Check sheet for the drawn part. Datum: minimum x, y, z corner. Units: mm. Round coordinates to 2 decimals unless told otherwise and drop trailing zeros. Order: outer loops, then holes, each group sorted by start corner. A loop starts at its lowest first (then second) coordinate and runs counter-clockwise, first axis right, second up. Notation, with made-up numbers: (-27, 49) -> (11, 49) arc R20 cw to (11, 66) -> close; hole circle Ø5 at (-29.5, 48). An arc over 180 degrees is marked (long way). Answer as a JSON object with one key per item and string values. Group by question number.
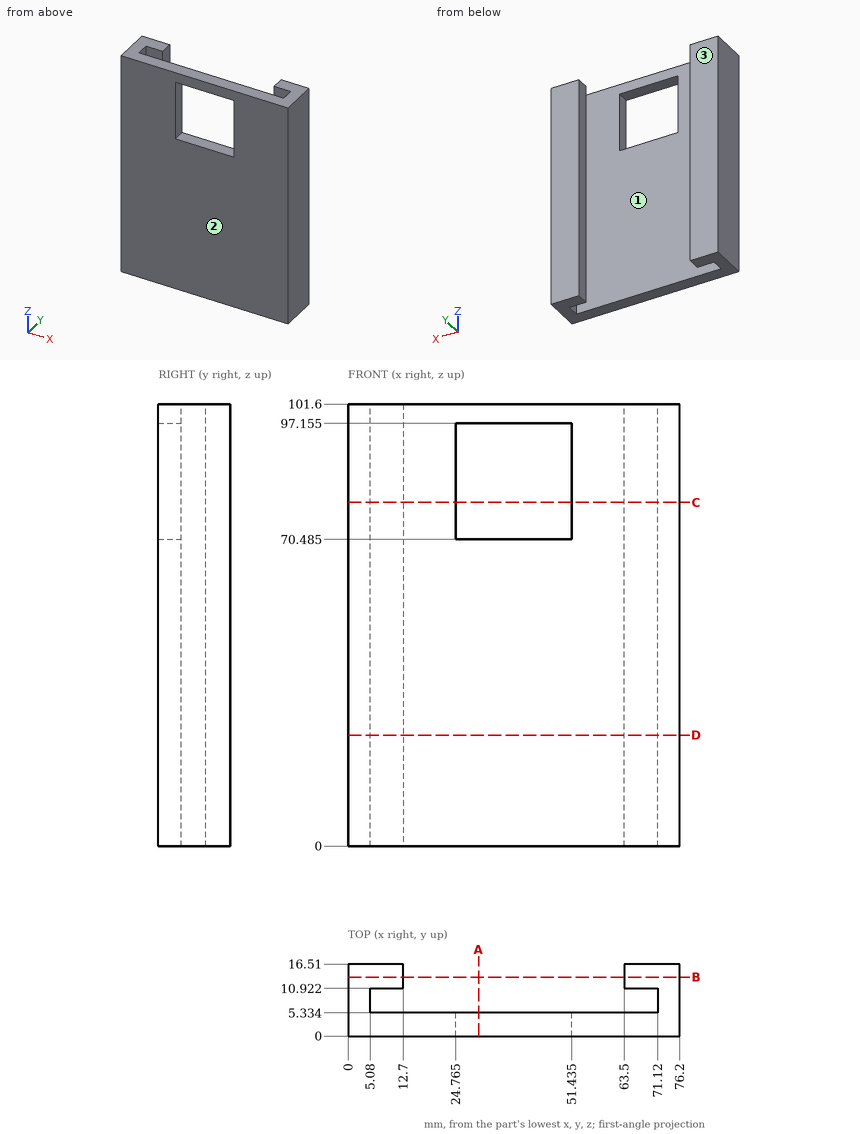
Item 1: Sectioned sample at D-D, the plane z = 25.5. Enter the section's corners in (x, y).
Item 2: Sectioned sample at A-A, the plane x = 30. Enter the section's corners in (y, z) (3 decimals).
Item 3: Depth check by flat-ended pin: pin 1 Ø1.5 at (x, y) = (14.5, 6.5) entering from +Z. Enter the tip coordinate at first touch or a pass-through.
Item 4: Mould release check, pull along Y, two halves, no side actions. Record for the marked faces 1, 2 and 3: pulls with the +Y half, pulls with the -Y half, needs draft (parallel to the pull), parting line crosses it, or undercut.
Item 5: Thickness scan on L1, parallel to X at y = 10.75, z = 73; L2, parallel to X at y = 15.5, z = 91; L3, parallel to Z at x = 27, y = 0.75 (3 decimals). Record the ranges inside material, lowest first.
Item 6: Sectioned sample at C-C, the plane z = 79. Enter the section's corners in (x, y) (3 decimals), then the cut area to 3 significant figures.
Item 7: Sectioned sample at B-B, the plane y = 13.5. Enter the section's corners in (x, z).
Result:
{
 "1": {"outline": "(0, 0) -> (76.2, 0) -> (76.2, 16.51) -> (63.5, 16.51) -> (63.5, 10.92) -> (71.12, 10.92) -> (71.12, 5.33) -> (5.08, 5.33) -> (5.08, 10.92) -> (12.7, 10.92) -> (12.7, 16.51) -> (0, 16.51) -> close"},
 "2": {"outline": "(0, 0) -> (5.334, 0) -> (5.334, 70.485) -> (0, 70.485) -> close; (0, 97.155) -> (5.334, 97.155) -> (5.334, 101.6) -> (0, 101.6) -> close"},
 "3": {"pin 1": "passes through"},
 "4": {"face 1": "undercut", "face 2": "pulls with the -Y half", "face 3": "pulls with the +Y half"},
 "5": {"L1": "x = 0 to 5.08, 71.12 to 76.2", "L2": "x = 0 to 12.7, 63.5 to 76.2", "L3": "z = 0 to 70.485, 97.155 to 101.6"},
 "6": {"outline": "(0, 0) -> (24.765, 0) -> (24.765, 5.334) -> (5.08, 5.334) -> (5.08, 10.922) -> (12.7, 10.922) -> (12.7, 16.51) -> (0, 16.51) -> close; (51.435, 0) -> (76.2, 0) -> (76.2, 16.51) -> (63.5, 16.51) -> (63.5, 10.922) -> (71.12, 10.922) -> (71.12, 5.334) -> (51.435, 5.334) -> close", "area": "463 mm2"},
 "7": {"outline": "(0, 0) -> (12.7, 0) -> (12.7, 101.6) -> (0, 101.6) -> close; (63.5, 0) -> (76.2, 0) -> (76.2, 101.6) -> (63.5, 101.6) -> close"}
}
